Geometry check sheet. Reference: the model listing, model coordinates, mm. Face numbers are marked on the shaded views. Give positions to 0.01 mm unless a question says otherwise; leave off trailing zeros. Order: outer loops, then holes, each group sorted by start corner. A loop starts at its lowest first (then second) coordinate and runs counter-clockwise, first axis right, second up.
```python
from build123d import *

# Parameters (mm, degrees)
BOSS_EXTRUDE1_DEPTH  = 6.35
M5_CLEARANCE_HOLE1_D = 5.5
M4_CLEARANCE_HOLE1_D = 4.5


with BuildPart() as part:
    # Sketch1 → Boss-Extrude1 (new body)
    with BuildSketch(Plane.XY):
        with BuildLine():
            Line((0, 6.35), (101.6, 6.35))
            ThreePointArc((101.6, 6.35), (107.95, 0), (101.6, -6.35))
            Line((101.6, -6.35), (0, -6.35))
            ThreePointArc((0, -6.35), (-6.35, 0), (0, 6.35))
        make_face()
    extrude(amount=BOSS_EXTRUDE1_DEPTH)

    # M5 Clearance Hole1 (through all)
    with Locations(Plane(origin=(0, 0, 0), x_dir=(-1, 0, 0), z_dir=(0, 0, -1))):
        with Locations((-101.6, 0)):
            Hole(M5_CLEARANCE_HOLE1_D / 2)

    # M4 Clearance Hole1 (through all)
    with Locations(Plane(origin=(0, 0, 0), x_dir=(-1, 0, 0), z_dir=(0, 0, -1))):
        with Locations((-50.8, 0), (0, 0)):
            Hole(M4_CLEARANCE_HOLE1_D / 2)


solid = part.part
```
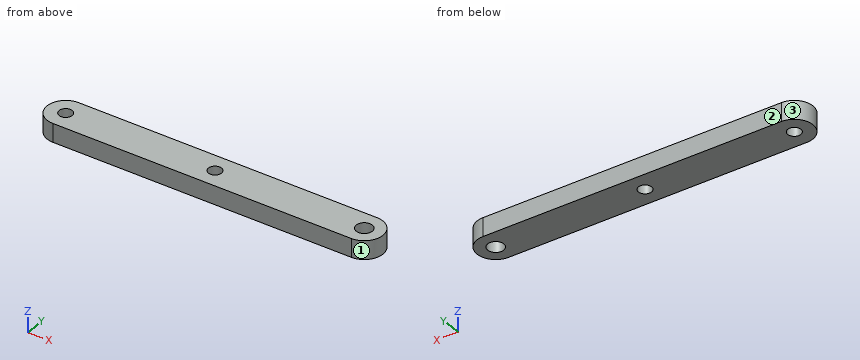
Q1. Thickness scan on L1, parallel to Y at x = 0, z = 1.5; L2, parallel to X at y = 1, z = 5; L3, parallel to Y at x = 101.6, z = 3.5. Record the ranges inside material, lowest first.
Q2. Cross-section at A-A, the plane y = 0. Record the boundary of the cut face in (x, z).
Q3. Cross-section at B-B, the plane z = 3.5. Record the boundary of the cut face in (x, y).
Q4. Gauge pin test, flat ends, axial feed: P1, Ø3.5, axis at x = 101.6, y = 0, coming from the +Z side; P2, Ø1.5, axis at x = 62.5, y = -4, coming from the -Z side. Record the tip position at first contact, or that the pin passes through.
Q5. Cross-section at D-D, the plane y = 4.25. Record the boundary of the cut face in (x, z), and give its area (3 significant figures).
Q6. Release check for a two-part mould opening along X. For the marked faces 1, 2 and 3 record: pulls with the +X half, pulls with the -X half, needs draft (parallel to the pull), parting line crosses it, or undercut.
Q7. Cross-section at C-C, the plane x = 50.8. Record the boundary of the cut face in (y, z).
Answers follow:
1. L1: y = -6.35 to -2.25, 2.25 to 6.35
1. L2: x = -6.27 to -2.02, 2.02 to 48.78, 52.82 to 99.04, 104.16 to 107.87
1. L3: y = -6.35 to -2.75, 2.75 to 6.35
2. outline: (-6.35, 0) - (-2.25, 0) - (-2.25, 6.35) - (-6.35, 6.35) - close; (2.25, 0) - (48.55, 0) - (48.55, 6.35) - (2.25, 6.35) - close; (53.05, 0) - (98.85, 0) - (98.85, 6.35) - (53.05, 6.35) - close; (104.35, 0) - (107.95, 0) - (107.95, 6.35) - (104.35, 6.35) - close
3. outline: (0, -6.35) - (101.6, -6.35) arc R6.35 ccw to (101.6, 6.35) - (0, 6.35) arc R6.35 ccw to start; hole circle Ø4.5 at (0, 0); hole circle Ø4.5 at (50.8, 0); hole circle Ø5.5 at (101.6, 0)
4. P1: passes through
4. P2: stops at z = 0
5. outline: (-4.72, 0) - (106.32, 0) - (106.32, 6.35) - (-4.72, 6.35) - close
5. area: 705 mm2
6. face 1: pulls with the +X half
6. face 2: needs draft
6. face 3: pulls with the -X half
7. outline: (-6.35, 0) - (-2.25, 0) - (-2.25, 6.35) - (-6.35, 6.35) - close; (2.25, 0) - (6.35, 0) - (6.35, 6.35) - (2.25, 6.35) - close
